Read the model definition and answer for the solid it produces. Units are mm, in the model's axes. A direction names the side the tool comes from. Coordinates: 2 decimals unless noted, no trailing zeros. Loops run counter-clockwise (first coordinate to the right, second up) from the corner with the lowest first, then second, coordinate; pieces in that order, holes last. Notation, with made-up numbers: (-35, -40) -> (1, -40) arc R28 cw to (1, -11) -> close; hole circle Ø9 at (13.5, 45.25). An arc over 180 degrees is marked (long way). Answer as a JSON object with one key per item and string values. Group by question number.
1) Section B-B, the plane x = -1 is taken. Give the vertices of the cut face in (y, z), plus the area to 3 significant figures.
2) Consider probe 1 along Z at (x, y) = (4.75, 1.25); probe 2 along X at (y, z) = (4.5, -0.75); probe 3 along Y at (x, z) = (3, -0.5). Determine where each line is inside the solid, lowest interval first. Write a range as [from, to].
3) Determine the mould class of faces 4 (the face through (0.4, 3.5, 1.5)), 5 (the face through (-6.6, 7.14, 0.05)), 6 (the face through (-0.1, 2, 1.5)) for opening direction Z: released by +Z, released by -Z, zero draft, split by the parting line, or undercut.
4) Flat-ended cylindrical pins translate along their axes: P1, Ø0.8, axis at x = -0.5, y = 3.5, coming from the +Z side; P2, Ø0.8, axis at x = 7.5, z = 3, coming from the +Y side; P3, Ø0.6, axis at x = 2, z = -2.5, coming from the +Y side; P4, Ø1, axis at x = 4, y = 8, coming from the -Z side. Find the tip coordinate at first contact, or state that the pin passes through.
5) Section C-C, the plane z = 3 is taken. Give the vertices of the cut face in (x, y), plus the area to 3 significant figures.
6) Which of the six approach directions +Z, -Z, +X, -X, +Y, -Y give full straight-line access (tool end or side, diameter ignored) to faces 1 (the face through (0, 1, -2)), 2 (the face through (1, 4, 0)), 3 (the face through (0.6, 3.5, -1.5))?
7) Section D-D, the plane y = 1 is taken. Give the vertices of the cut face in (x, z).
8) Section A-A, the plane y = 4.5 is taken. Give the vertices of the cut face in (x, z).
Autodesk Fusion 360 part; units mm, degrees
sketch "Sketch1" plane through (0, 0, 0) normal (1, 0, 0) x (0, 0, -1)
sketch "Sketch1 (2)" plane through (0, 0, 0) normal (0, 1, 0) x (1, 0, 0) in component "Component"
  line L0 (8.5, -3.5) -> (-8.5, -3.5)
  line L1 (-8.5, -3.5) -> (-8.5, 3.5)
  line L2 (-8.5, 3.5) -> (8.5, 3.5)
  line L3 (8.5, 3.5) -> (8.5, -3.5)
  line L4 (8.5, -3.5) -> (-8.5, 3.5) construction
  line L5 (-8.5, -3.5) -> (8.5, 3.5) construction
  dimension "d1" = 17
  dimension "d2" = 7
extrude "Extrude1" add sketch "Sketch1 (2)" along normal blind 5 in component "Component"
sketch "Sketch2" plane through (-8.5, 0, 0) normal (-1, 0, 0) x (0, 0, 1) in component "Component"
  line L0 (-3.5, 0) -> (3.5, 0)
  line L1 (3.5, 0) -> (3.5, 5)
  line L2 (3.5, 5) -> (-3.5, 5)
  line L3 (-3.5, 5) -> (-3.5, 0)
  line L4 (-2, 0) -> (-2, 2)
  line L5 (-2, 2) -> (-1, 2)
  line L6 (-1, 2) -> (-1, 3.5)
  line L7 (-1, 3.5) -> (1, 3.5)
  line L8 (1, 3.5) -> (1, 2)
  line L9 (1, 2) -> (2, 2)
  line L10 (2, 2) -> (2, 0)
extrude "Extrude2" cut sketch "Sketch2" against normal up to surface (17 mm away) contours L0 L4 L5 L6 L7 L8 L9 L10 in component "Component"
sketch "Sketch3" plane through (0, 0, 3.5) normal (0, 0, 1) x (1, 0, 0) in component "Component"
  line L0 (-8.5, 0) -> (8.5, 0)
  line L1 (8.5, 0) -> (8.5, 5)
  line L2 (8.5, 5) -> (-8.5, 5)
  line L3 (-8.5, 5) -> (-8.5, 0)
  circle A0 centre (-4.5, 5) radius 3
  line L4 (-4.5, 5) -> (-4.5, 8)
extrude "Extrude3" add sketch "Sketch3" against normal up to surface (7 mm away) contours L2 A0 L4 picked at (-5.6955, 6.597) in component "Component"
sketch "Sketch4" plane through (0, 5, 0) normal (0, 1, 0) x (-1, 0, 0) in component "Component"
  line L0 (4.5, -3.5) -> (4.5, 3.5)
  line L1 (4.5, 3.5) -> (-8.5, 3.5)
  line L2 (-8.5, 3.5) -> (-8.5, -3.5)
  line L3 (-8.5, -3.5) -> (4.5, -3.5)
  line L4 (-5.5, -3.5) -> (-5.5, 3.5)
extrude "Extrude4" add sketch "Sketch4" along normal blind 2 contours L1 L2 L3 L4 in component "Component"
sketch "Sketch5" plane through (8.5, 0, 0) normal (1, 0, 0) x (0, 0, -1) in component "Component"
  line L0 (-2, 0) -> (-2, 2)
  line L1 (-2, 2) -> (-1, 2)
  line L2 (-1, 2) -> (-1, 3.5)
  line L3 (-1, 3.5) -> (1, 3.5)
  line L4 (1, 3.5) -> (1, 2)
  line L5 (1, 2) -> (2, 2)
  line L6 (2, 2) -> (2, 0)
  line L7 (2, 0) -> (3.5, 0)
  line L8 (3.5, 0) -> (3.5, 7)
  line L9 (3.5, 7) -> (-3.5, 7)
  line L10 (-3.5, 7) -> (-3.5, 0)
  line L11 (-3.5, 0) -> (-2, 0)
  circle A0 centre (0, 7) radius 2
extrude "Extrude5" add sketch "Sketch5" against normal up to surface (3 mm away) contours L9 A0 picked at (0.4157, 7.5212) in component "Component"
sketch "Sketch6" plane through (0, 0, 3.5) normal (0, 0, 1) x (1, 0, 0) in component "Component"
  line L0 (-8.5, 0) -> (8.5, 0)
  line L1 (8.5, 0) -> (8.5, 7)
  line L2 (8.5, 7) -> (5.5, 7)
  line L3 (5.5, 7) -> (5.5, 5)
  line L4 (5.5, 5) -> (-4.5, 5)
  line L5 (-4.5, 5) -> (-4.5, 8)
  arc A0 (-4.5, 8) -> (-7.5, 5) centre (-4.5, 5) ccw
  line L6 (-7.5, 5) -> (-8.5, 5)
  line L7 (-8.5, 5) -> (-8.5, 0)
  line L8 (-4.5, 3) -> (5.5, 3)
  line L9 (5.5, 3) -> (5.5, 5)
  line L10 (-4.5, 3) -> (-4.5, 3.127)
  line L11 (-4.5, 3.127) -> (-4.5, 5)
extrude "Extrude6" cut sketch "Sketch6" against normal blind 2 contours L4 L8 L9 L10 L11 in component "Component"
sketch "Sketch7" plane through (0, 0, -3.5) normal (0, 0, -1) x (-1, 0, 0) in component "Component"
  line L0 (-8.5, 0) -> (8.5, 0)
  line L1 (8.5, 0) -> (8.5, 5)
  line L2 (8.5, 5) -> (7.5, 5)
  arc A0 (7.5, 5) -> (4.5, 8) centre (4.5, 5) ccw
  line L3 (4.5, 8) -> (4.5, 5)
  line L4 (4.5, 5) -> (-5.5, 5)
  line L5 (-5.5, 5) -> (-5.5, 7)
  line L6 (-5.5, 7) -> (-8.5, 7)
  line L7 (-8.5, 7) -> (-8.5, 0)
  line L8 (-5.5, 3) -> (4.5, 3)
  line L9 (4.5, 3) -> (4.5, 5)
  line L10 (-5.5, 3) -> (-5.5, 5)
extrude "Extrude7" cut sketch "Sketch7" against normal blind 2 contours L4 L8 L9 L10 in component "Component"
sketch "Sketch8" plane through (0, 5, 0) normal (0, 1, 0) x (-1, 0, 0) in component "Component"
  line L0 (-5.5, -1.5) -> (4.5, -1.5)
  line L1 (4.5, -1.5) -> (4.5, 1.5)
  line L2 (4.5, 1.5) -> (-5.5, 1.5)
  line L3 (-5.5, 1.5) -> (-5.5, -1.5)
extrude "Extrude8" cut sketch "Sketch8" against normal blind 1 in component "Component"
component "Component" placed x (1, 0, 0) y (0, 1, 0) z (0, 0, 1) at (0, 0, 0)
Determined:
{
 "1": {"outline": "(0, -3.5) -> (3, -3.5) -> (3, -1.5) -> (4, -1.5) -> (4, 1.5) -> (3, 1.5) -> (3, 3.5) -> (0, 3.5) -> (0, 2) -> (2, 2) -> (2, 1) -> (3.5, 1) -> (3.5, -1) -> (2, -1) -> (2, -2) -> (0, -2) -> close", "area": "13.0 mm²"},
 "2": {"probe 1": "[-3.5, -2], [2, 3.5]", "probe 2": "[-8.5, -4.5], [5.5, 8.5]", "probe 3": "[3.5, 4]"},
 "3": {"face 4": "released by +Z", "face 5": "zero draft", "face 6": "undercut"},
 "4": {"P1": "z = 1.5", "P2": "y = 7", "P3": "y = 3", "P4": "through"},
 "5": {"outline": "(-8.5, 0) -> (8.5, 0) -> (8.5, 7) -> (5.5, 7) -> (5.5, 3) -> (-4.5, 3) -> (-4.5, 8) arc R3 ccw to (-7.5, 5) -> (-8.5, 5) -> close", "area": "78.1 mm²"},
 "6": {"face 1": "+X, -X, -Y", "face 2": "+Z, -Z, +Y", "face 3": "-Z, +Y"},
 "7": {"outline": "(-8.5, -3.5) -> (8.5, -3.5) -> (8.5, -2) -> (-8.5, -2) -> close; (-8.5, 2) -> (8.5, 2) -> (8.5, 3.5) -> (-8.5, 3.5) -> close"},
 "8": {"outline": "(-8.5, -3.5) -> (-4.5, -3.5) -> (-4.5, 3.5) -> (-8.5, 3.5) -> close; (5.5, -3.5) -> (8.5, -3.5) -> (8.5, 3.5) -> (5.5, 3.5) -> close"}
}
